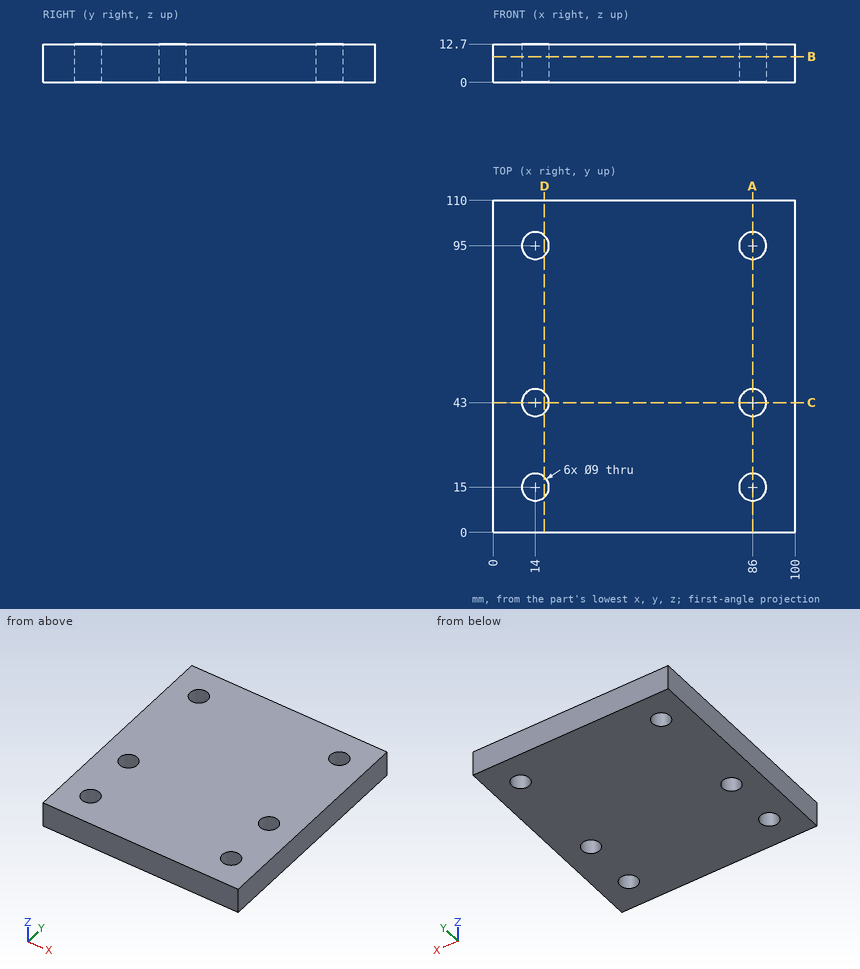
Input: dimensioned drawing with shaded views. Units: mm. Origin: part minimum x, y, z. Coordinates: 2 decimals unless noted, no trailing zeros. Write each loop counter-clockwise with the first axis right and the second up, starting at its lowest first coordinate (ties: lowest second). Pieces come first, ordered by that corner, then holes. Notation, with made-up numbers: M -25.5,3 L 21.5,3 A18 cw 21.5,19 Z; hole C 18.5,-1 d11. An arc over 180 degrees is marked long. Answer as a JSON object with one key per item and string values. Group by question number.
(1) Contact query for flat-ended pins moving along their axis: P1, Ø5.5, axis at x = 14, y = 15, coming from the +Z side; P2, Ø14.5, axis at x = 14, y = 95, coming from the -Z side. Output: stop coordinate, or through.
(2) Section C-C on y = 43. Output: boundary loops of the cut face in (x, z).
(3) Section B-B on z = 8.5. Output: boundary loops of the cut face in (x, y), plus the area to 3 significant figures.
(4) Section A-A on x = 86. Output: boundary loops of the cut face in (y, z), plus the area to 3 significant figures.
(5) Section D-D on x = 17. Output: boundary loops of the cut face in (y, z).
(6) Ray query, line 1 along X through (y, z) = (43, 5.5); line 2 along Y through (x, z) = (14, 4.75); line 3 along X through (y, z) = (47, 8.5). Return the intervals inside material, ascending. Write a range as [from, to].
Result set:
{
 "1": {"P1": "passes through", "P2": "stops at z = 0"},
 "2": {"outline": "M 0,0 L 9.5,0 L 9.5,12.7 L 0,12.7 Z; M 18.5,0 L 81.5,0 L 81.5,12.7 L 18.5,12.7 Z; M 90.5,0 L 100,0 L 100,12.7 L 90.5,12.7 Z"},
 "3": {"outline": "M 0,0 L 100,0 L 100,110 L 0,110 Z; hole C 14,15 d9; hole C 14,43 d9; hole C 14,95 d9; hole C 86,15 d9; hole C 86,43 d9; hole C 86,95 d9", "area": "10,600 mm2"},
 "4": {"outline": "M 0,0 L 10.5,0 L 10.5,12.7 L 0,12.7 Z; M 19.5,0 L 38.5,0 L 38.5,12.7 L 19.5,12.7 Z; M 47.5,0 L 90.5,0 L 90.5,12.7 L 47.5,12.7 Z; M 99.5,0 L 110,0 L 110,12.7 L 99.5,12.7 Z", "area": "1,050 mm2"},
 "5": {"outline": "M 0,0 L 11.65,0 L 11.65,12.7 L 0,12.7 Z; M 18.35,0 L 39.65,0 L 39.65,12.7 L 18.35,12.7 Z; M 46.35,0 L 91.65,0 L 91.65,12.7 L 46.35,12.7 Z; M 98.35,0 L 110,0 L 110,12.7 L 98.35,12.7 Z"},
 "6": {"line 1": "x = [0, 9.5], [18.5, 81.5], [90.5, 100]", "line 2": "y = [0, 10.5], [19.5, 38.5], [47.5, 90.5], [99.5, 110]", "line 3": "x = [0, 11.94], [16.06, 83.94], [88.06, 100]"}
}
